from build123d import *

# Parameters (mm, degrees)
SKETCH1_R         = 1.46
SKETCH2_R         = 1
DOME1_FACE_RADIUS = 1.46
DOME1_HEIGHT      = 1.46


with BuildPart() as part:
    # Sketch1 → Loft1 section 0
    with BuildSketch(Plane(origin=(0, 0, 0), x_dir=(1, 0, 0), z_dir=(0, 1, 0))):
        Circle(SKETCH1_R)
    # Sketch2 → Loft1 section 1
    with BuildSketch(Plane(origin=(0, -12, 0), x_dir=(1, 0, 0), z_dir=(0, 1, 0))):
        Circle(SKETCH2_R)
    loft()

    # Dome1: a dome of height H over a round flat face of radius A is a cap of a sphere of radius (A * A + H * H) / (2 * H)
    dome1_r = (DOME1_FACE_RADIUS * DOME1_FACE_RADIUS + DOME1_HEIGHT * DOME1_HEIGHT) / (2 * DOME1_HEIGHT)
    dome1_base = Plane((0, 0, 0), z_dir=(0, 1, 0))
    with Locations(dome1_base.offset(DOME1_HEIGHT - dome1_r)):
        dome1_ball = Sphere(dome1_r, mode=Mode.PRIVATE)
    add(split(dome1_ball, bisect_by=dome1_base, keep=Keep.TOP, mode=Mode.PRIVATE))

    # Sketch3 → Revolve3 (revolve)
    with BuildSketch(Plane.XY, mode=Mode.PRIVATE) as revolve3_sk:
        with BuildLine():
            Line((0, -12), (0, -14.236067977))
            Line((0, -14.236067977), (1, -14.236067977))
            ThreePointArc((1, -14.236067977), (1.5, -13.118033989), (1, -12))
            Line((1, -12), (0, -12))
        make_face()
    revolve(revolve3_sk.sketch.rotate(Axis((0, -12, 0), (0, -1, 0)), 270), axis=Axis((0, -12, 0), (0, -1, 0)))


solid = part.part
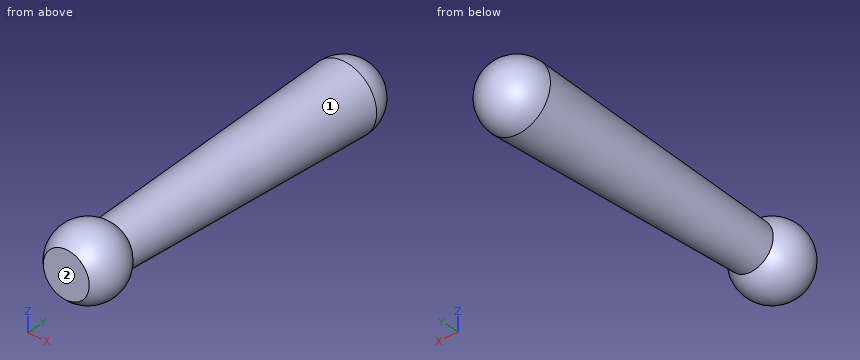
Geometry: final body of the model. Coordinates: model frame, mm. Face numbers are marked on the shaded views. Give positions to 0.01 mm unless a question says otherwise; leave off trailing zeros. Write each loop counter-clockwise with the first axis right and the second up, starting at its lowest first coordinate (ties: lowest second). Pieces come first, ordered by that corner, then holes. Notation, with made-up numbers: (14.25, 64) -> (43.25, 64) arc R12 ccw to (43.25, 77) -> close; hole circle Ø3 at (5.25, -34.5). An arc over 180 degrees is marked (long way). Answer in a Markdown table with one row per item.
(1) Ray query, line 1 along Z through (x, y) = (1.1, -3.5); line 2 along Z through (x, y) = (0.55, -6.25); line 3 along X through (y, z) = (-13, -0.75). Return the intervals inside material, ascending. Write a range as [from, to].
Answers below:
| item | result |
|---|---|
| line 1 | [-0.74, 0.74] |
| line 2 | [-1.09, 1.09] |
| line 3 | [-1.29, 1.29] |
(2) Draft query along Y for the marked faces 1 and 2. Return one class per face: +Y half, -Y half, draft (parallel to the pull), parting line (faces both ways), or undercut.
Answers below:
| item | result |
|---|---|
| face 1 | undercut |
| face 2 | -Y half |
(3) Section query A-A on x = 0. Return loops of the section in (y, z), then the cut area to 3 significant figures.
Answers below:
| item | result |
|---|---|
| outline | (-14.24, -1) arc R1.5 ccw to (-12, -1) -> (0, -1.46) arc R1.46 ccw to (0, 1.46) -> (-12, 1) arc R1.5 ccw to (-14.24, 1) -> close |
| area | 38.9 mm^2 |
(4) Pin query (flat end, axial travel): pin 1 (1.5 mm diameter, centred on x = -0.5, z = -1, fed in from +Y); pin 2 (1.5 mm diameter, centred on y = -6, z = -1, fed in from +X). Return the tip coordinate at first contact, or that it passes through.
Answers below:
| item | result |
|---|---|
| pin 1 | y = 1.41 |
| pin 2 | x = 1.21 |
(5) Section query B-B on y = -9.5. Return loops of the section in (x, z), then the cut area to 3 significant figures.
Answers below:
| item | result |
|---|---|
| outline | circle Ø2.19 at (0, 0) |
| area | 3.77 mm^2 |
(6) Section query C-C on y = -3.75. Return loops of the section in (x, z).
Answers below:
| item | result |
|---|---|
| outline | circle Ø2.63 at (0, 0) |
